Verification items for the finished model (mm, model axes). Face numbers are marked on the shaded views. A direction names the side the tool comes from. Coordinates: 2 decimals unless noted, no trailing zeros. Loops run counter-clockwise (first coordinate to the right, second up) from the corner with the lowest first, then second, coordinate; pieces in that order, holes last.
Q1. Go/stop test with flat-tipped pins: P1, Ø1.5, axis at x = 15.5, y = 3.5, coming from the -Z side; P2, Ø8, axis at x = 12.5, z = 5.5, coming from the -Y side; P3, Ø6, axis at x = 17.5, z = -4, coming from the -Y side. Record where each tip stops, or that it passes through.
Q2. Sectioned sample at C-C (z = 6.5). Enter the section's corners in (x, y).
Q3. Material ranges on probe 1 along X at (y, z) = (-5, 5.25); probe 2 along Z at (x, y) = (22.3, 0); probe 3 along Z at (x, y) = (0, 0), recorded low to high.
Q4. Access from +Z, -Z, +X, -X, +Y, -Y to the whole of each face (thin tool, end or side, straight path). Record for the marked faces 4 and 5.
Q5. Sectioned sample at B-B (x = 2). Enter the section's corners in (y, z).
Q6. Mould release check, pull along Z, two halves, no side actions. Record for the marked faces 1, 2 and 3: +Z half, -Z half, draft (parallel to the pull), parting line (faces both ways), or undercut.
Q7. Sectioned sample at A-A (y = -5.75). Enter the section's corners in (x, z).
```python
from build123d import *

# Parameters (mm, degrees)
F0_R      = 7.5
F0_R_2    = 4
F1_DEPTH  = 22.5
F4_R      = 8
F4_R_2    = 7.15
F5_DEPTH  = 1.1
F6_R      = 8
F6_R_2    = 7.15
F7_DEPTH  = 1.1
F8_R      = 7.15
F8_R_2    = 4.35
F9_DEPTH  = 0.5
F11_R     = 7.15
F11_R_2   = 4.35
F12_DEPTH = 0.5


with BuildPart() as f1:
    # F0 (on Right) → F1 (new body, symmetric)
    with BuildSketch(Plane.YZ):
        Circle(F0_R)
        Circle(F0_R_2, mode=Mode.SUBTRACT)
    extrude(amount=F1_DEPTH, both=True)

    # F4 (on offset) → F5 (cut)
    with BuildSketch(Plane.YZ.offset(-17.5)):
        Circle(F4_R)
        Circle(F4_R_2, mode=Mode.SUBTRACT)
    extrude(amount=F5_DEPTH, mode=Mode.SUBTRACT)

    # F6 (on offset) → F7 (cut)
    with BuildSketch(Plane.YZ.offset(17.5)):
        Circle(F6_R)
        Circle(F6_R_2, mode=Mode.SUBTRACT)
    extrude(amount=-F7_DEPTH, mode=Mode.SUBTRACT)

    # F8 (on face) → F9 (cut)
    with BuildSketch(Plane.YZ.offset(22.5)):
        Circle(F8_R)
        Circle(F8_R_2, mode=Mode.SUBTRACT)
    extrude(amount=-F9_DEPTH, mode=Mode.SUBTRACT)

    # F11 (on face) → F12 (cut)
    with BuildSketch(Plane(origin=(-22.5, 0, 0), x_dir=(0, -1, 0), z_dir=(-1, 0, 0))):
        Circle(F11_R)
        Circle(F11_R_2, mode=Mode.SUBTRACT)
    extrude(amount=-F12_DEPTH, mode=Mode.SUBTRACT)


solid = f1.part
```
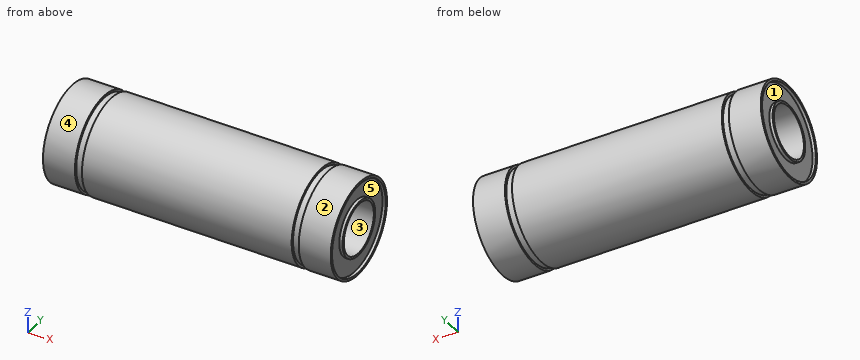
Geometry check:
1. P1: stops at z = -6.98
1. P2: stops at y = -7.35
1. P3: stops at y = -7.43
2. outline: (-22.5, -3.74) - (-17.5, -3.74) - (-17.5, -2.98) - (-16.4, -2.98) - (-16.4, -3.74) - (16.4, -3.74) - (16.4, -2.98) - (17.5, -2.98) - (17.5, -3.74) - (22.5, -3.74) - (22.5, -2.98) - (22, -2.98) - (22, 2.98) - (22.5, 2.98) - (22.5, 3.74) - (17.5, 3.74) - (17.5, 2.98) - (16.4, 2.98) - (16.4, 3.74) - (-16.4, 3.74) - (-16.4, 2.98) - (-17.5, 2.98) - (-17.5, 3.74) - (-22.5, 3.74) - (-22.5, 2.98) - (-22, 2.98) - (-22, -2.98) - (-22.5, -2.98) - close
3. probe 1: x = -22.5 to -17.5, -16.4 to 16.4, 17.5 to 22.5
3. probe 2: z = -7.5 to -7.15, -4.35 to -4, 4 to 4.35, 7.15 to 7.5
3. probe 3: z = -7.5 to -4, 4 to 7.5
4. face 4: +X, -X
4. face 5: +X
5. outline: circle Ø15 at (0, 0); hole circle Ø8 at (0, 0)
6. face 1: undercut
6. face 2: parting line
6. face 3: undercut
7. outline: (-22.5, -4.82) - (-17.5, -4.82) - (-17.5, -4.25) - (-16.4, -4.25) - (-16.4, -4.82) - (16.4, -4.82) - (16.4, -4.25) - (17.5, -4.25) - (17.5, -4.82) - (22.5, -4.82) - (22.5, -4.25) - (22, -4.25) - (22, 4.25) - (22.5, 4.25) - (22.5, 4.82) - (17.5, 4.82) - (17.5, 4.25) - (16.4, 4.25) - (16.4, 4.82) - (-16.4, 4.82) - (-16.4, 4.25) - (-17.5, 4.25) - (-17.5, 4.82) - (-22.5, 4.82) - (-22.5, 4.25) - (-22, 4.25) - (-22, -4.25) - (-22.5, -4.25) - close
